Verification items for the finished model (mm, model axes). Face numbers are marked on the shaded views. A direction names the side the tool comes from. Round coordinates to 2 decimals unless told otherwise and drop trailing zeros. Write each loop counter-clockwise with the first axis right and the second up, starting at its lowest first coordinate (ties: lowest second). Pieces come first, ordered by that corner, then holes. Notation, with made-up numbers: (11.5, 70.5) - (40.5, 70.5) arc R23 ccw to (40.5, 89.5) - close; hole circle Ø7 at (43.25, 35.25). An arc over 180 degrees is marked (long way). Answer as a JSON object with one key per item and string values.
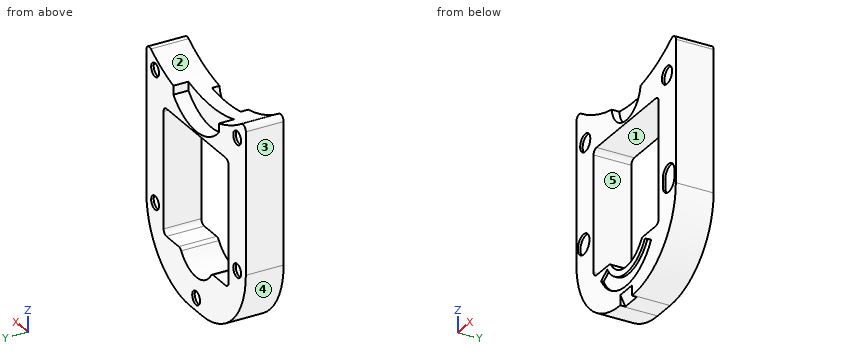
```python
from build123d import *

# Parameters (mm, degrees)
BASE_DEPTH                      = 38.1
SKETCH2_R                       = 8.89
SKETCH2_R_2                     = 10.16
COFFEE_MAKER_FEET_CUTOUTS_DEPTH = 2.54
ASYMMETRIC_FOOT_SLOT_DEPTH      = 2.54
FRONT_START                     = -38.1
SKETCH11_R                      = 25.4
FRONT_CUTOUT_DEPTH              = 7.62
FILLET1_R                       = 76.2
DRIP_START                      = -38.1
DRIP_TRAY_CUTOUT_DEPTH          = 15.24
SKETCH5_R                       = 6.858
FEET_PADS_DEPTH                 = 2.54
CENTER_CUTOUT_DEPTH             = 221.978403371
FILLET2_R                       = 5.08
FILLET4_R                       = 5.08
EASY_PRINTER_RELEASE_TAB_DEPTH  = 10.16


with BuildPart() as part:
    # Sketch1 → Base (new body)
    with BuildSketch(Plane(origin=(0, 0, 0), x_dir=(1, 0, 0), z_dir=(0, 1, 0))):
        with BuildLine():
            Line((-87.3125, 199.39), (-87.3125, -29.21))
            ThreePointArc((-87.3125, -29.21), (0, 0), (87.3125, -29.21))
            Line((87.3125, -29.21), (87.3125, 199.39))
            Line((87.3125, 199.39), (-87.3125, 199.39))
        make_face()
    extrude(amount=BASE_DEPTH)

    # Sketch2 → Coffee Maker Feet Cutouts (cut)
    with BuildSketch(Plane(origin=(0, 0, 0), x_dir=(-1, 0, 0), z_dir=(0, -1, 0))):
        with Locations(Location((71.834375, 8.89, 0), (0, 0, 90))):
            Circle(SKETCH2_R)
        with Locations(Location((74.549, 108.712, 0), (0, 0, 90))):
            Circle(SKETCH2_R_2)
        with Locations(Location((-74.549, 108.712, 0), (0, 0, 90))):
            Circle(SKETCH2_R_2)
        with Locations(Location((-71.834375, 8.89, 0), (0, 0, 90))):
            Circle(SKETCH2_R)
        with BuildLine():
            Line((-43.994090512, 159.512), (-32.995567884, 153.162))
            ThreePointArc((-32.995567884, 153.162), (0, 172.212), (32.995567884, 153.162))
            Line((32.995567884, 153.162), (43.994090512, 159.512))
            ThreePointArc((43.994090512, 159.512), (0, 184.912), (-43.994090512, 159.512))
        make_face()
    extrude(amount=-COFFEE_MAKER_FEET_CUTOUTS_DEPTH, mode=Mode.SUBTRACT)

    # Sketch10 → Asymmetric Foot Slot (cut)
    with BuildSketch(Plane(origin=(0, 0, 0), x_dir=(-1, 0, 0), z_dir=(0, -1, 0))):
        with BuildLine():
            Line((-84.709, 108.712), (-84.709, 116.332))
            ThreePointArc((-84.709, 116.332), (-74.549, 126.492), (-64.389, 116.332))
            Line((-64.389, 116.332), (-64.389, 108.712))
            ThreePointArc((-64.389, 108.712), (-74.549, 98.552), (-84.709, 108.712))
        make_face()
    extrude(amount=-ASYMMETRIC_FOOT_SLOT_DEPTH, mode=Mode.SUBTRACT)

    # Sketch11 → Front cutout (cut)
    with BuildSketch(Plane(origin=(0, 38.1, 0), x_dir=(1, 0, 0), z_dir=(0, 1, 0)).offset(FRONT_START)):
        with Locations((0, -5.08)):
            Circle(SKETCH11_R)
    extrude(amount=FRONT_CUTOUT_DEPTH, mode=Mode.SUBTRACT)

    # Fillet1
    fillet1_edges = [part.edges().sort_by_distance(p)[0] for p in [
        (87.3125, 19.05, -199.39),
        (-87.3125, 19.05, -199.39),
    ]]
    fillet(fillet1_edges, radius=FILLET1_R)

    # Sketch4 → Drip Tray Cutout (cut)
    with BuildSketch(Plane.XZ.offset(DRIP_START)):
        with BuildLine():
            Line((40.005, -3.26616737), (40.005, 5.62383263))
            Line((40.005, 5.62383263), (-40.005, 5.62383263))
            Line((-40.005, 5.62383263), (-40.005, -3.26616737))
            ThreePointArc((-40.005, -3.26616737), (0, -21.04616737), (40.005, -3.26616737))
        make_face()
    extrude(amount=DRIP_TRAY_CUTOUT_DEPTH, mode=Mode.SUBTRACT)

    # Sketch5 → Feet Pads (cut)
    with BuildSketch(Plane(origin=(0, 38.1, 0), x_dir=(1, 0, 0), z_dir=(0, 1, 0))):
        with Locations(Location((-72.0725, -6.35, 0), (0, 0, 270))):
            Circle(SKETCH5_R)
        with Locations(Location((-72.0725, 125.73, 0), (0, 0, 270))):
            Circle(SKETCH5_R)
        with Locations(Location((0, 186.69, 0), (0, 0, 270))):
            Circle(SKETCH5_R)
        with Locations(Location((72.0725, 125.73, 0), (0, 0, 90))):
            Circle(SKETCH5_R)
        with Locations(Location((72.0725, -6.35, 0), (0, 0, 90))):
            Circle(SKETCH5_R)
    extrude(amount=-FEET_PADS_DEPTH, mode=Mode.SUBTRACT)

    # Sketch6 → Center cutout (cut, through all)
    with BuildSketch(Plane(origin=(0, 0, 0), x_dir=(-1, 0, 0), z_dir=(0, -1, 0))):
        with BuildLine():
            Line((27.569240033, 149.86), (57.15, 149.86))
            Line((57.15, 149.86), (57.15, 22.86))
            Line((57.15, 22.86), (-57.15, 22.86))
            Line((-57.15, 22.86), (-57.15, 149.86))
            Line((-57.15, 149.86), (-27.569240033, 149.86))
            ThreePointArc((-27.569240033, 149.86), (0, 165.862), (27.569240033, 149.86))
        make_face()
    extrude(amount=-CENTER_CUTOUT_DEPTH, mode=Mode.SUBTRACT)

    # Fillet2
    fillet2_edges = [part.edges().sort_by_distance(p)[0] for p in [
        (57.15, 19.05, -22.86),
        (57.15, 19.05, -149.86),
        (27.569240033, 19.05, -149.86),
        (-27.569240033, 19.05, -149.86),
        (-57.15, 19.05, -149.86),
        (-57.15, 19.05, -22.86),
    ]]
    fillet(fillet2_edges, radius=FILLET2_R)

    # Fillet4
    fillet4_edges = [part.edges().sort_by_distance(p)[0] for p in [
        (87.3125, 19.05, 29.21),
        (-87.3125, 19.05, 29.21),
    ]]
    fillet(fillet4_edges, radius=FILLET4_R)

    # Sketch9 → Easy-Printer-Release-Tab (cut, symmetric)
    with BuildSketch(Plane(origin=(0, 0, 0), x_dir=(0, 0, -1), z_dir=(1, 0, 0))):
        Polygon((199.39, 5.08), (189.23, 0), (199.39, 0), align=None)
    extrude(amount=EASY_PRINTER_RELEASE_TAB_DEPTH, both=True, mode=Mode.SUBTRACT)


solid = part.part
```
Q1. Section check A-A, the plane z = -66.5. Record the cut outline in (x, y).
Geometry check:
{"outline": "(-87.31, 0) - (-57.15, 0) - (-57.15, 38.1) - (-87.31, 38.1) - close; (57.15, 0) - (87.31, 0) - (87.31, 38.1) - (57.15, 38.1) - close"}
Q2. Gauge pin test, flat ends, axial feed: P1, Ø4, axis at x = -73.5, z = -124.5, coming from the +Y side; P2, Ø6, axis at x = 15, y = 14, coming from the -Z side; P3, Ø2, axis at x = -49, y = 4.5, coming from the +Z side. Record the tip position at first contact, or that the pin passes through.
Geometry check:
{"P1": "stops at y = 35.56", "P2": "stops at z = -199.38", "P3": "stops at z = 8.89"}
Q3. Set-up check for the marked faces 1 and 2: record each of +Z, -Z, +X, -X, +Y, -Y from which the full face is reachable in a straight line by a thin tool's end or side.
Geometry check:
{"face 1": "+Y, -Y", "face 2": "+Z, +Y, -Y"}
Q4. Section check B-B, the plane x = 0. Record the cut outline in (y, z).
Geometry check:
{"outline": "(0, -189.23) - (5.08, -199.39) - (38.1, -199.39) - (38.1, -193.55) - (35.56, -193.55) - (35.56, -179.83) - (38.1, -179.83) - (38.1, -165.86) - (0, -165.86) - (0, -172.21) - (2.54, -172.21) - (2.54, -184.91) - (0, -184.91) - close; (0, -22.86) - (38.1, -22.86) - (38.1, -21.05) - (22.86, -21.05) - (22.86, 0) - (7.62, 0) - (7.62, -20.32) - (0, -20.32) - close"}
Q5. Section check D-D, the plane z = -8.89. Record the cut outline in (x, y), then the cut area to 3 significant figures.
Geometry check:
{"outline": "(-87.31, 0) - (-80.72, 0) - (-80.72, 2.54) - (-62.94, 2.54) - (-62.94, 0) - (-21.21, 0) - (-21.21, 7.62) - (21.21, 7.62) - (21.21, 0) - (62.94, 0) - (62.94, 2.54) - (80.72, 2.54) - (80.72, 0) - (87.31, 0) - (87.31, 38.1) - (34.1, 38.1) - (34.1, 22.86) - (-34.1, 22.86) - (-34.1, 38.1) - (-87.31, 38.1) - close", "area": "5,200 mm2"}
Q6. Release check for a two-part mould opening along Z. For the marked faces 3, 4 and 5 record: released by +Z, released by -Z, zero draft, split by the parting line, or undercut.
Geometry check:
{"face 3": "zero draft", "face 4": "released by -Z", "face 5": "undercut"}
Q7. Material ranges on line 1 along X through (y, z) = (26, -94); line 2 along Y through (x, z) = (80.5, -109.5); line 3 along X through (y, z) = (1.15, -8.89), recorded low to high. Write a range as [from, to].
Geometry check:
{"line 1": "x = [-87.31, -57.15], [57.15, 87.31]", "line 2": "y = [2.54, 38.1]", "line 3": "x = [-87.31, -80.72], [-62.94, -21.21], [21.21, 62.94], [80.72, 87.31]"}
